Verification items for the finished model (mm, model axes). A direction names the side the tool comes from. Round coordinates to 2 decimals unless told otherwise and drop trailing zeros. Order: outer loops, then holes, each group sorted by start corner. A loop starts at its lowest first (then second) coordinate and runs counter-clockwise, first axis right, second up. Notation, with made-up numbers: (-31, 89) -> (6, 89) arc R11 ccw to (6, 107) -> close; hole circle Ø3 at (26, 63). An arc over 180 degrees is marked (long way). Return JSON: item names as keys, results as strings. Group by question number.
Item 1: Sectioned sample at C-C on z = 11. Record the cut outline in (x, y).
Item 2: Draft check along X on faces 5 (the flat face through (21.431, 0, 0)), 6 (the conical face through (0.16, 1.08, -0.71)), 7 (the cylindrical face through (-8.798, 9.296, -0.133)). Enter one of: pulls with the +X half, pulls with the -X half, needs draft (parallel to the pull), parting line crosses it, or undercut.
Item 3: Sectioned sample at B-B on y = 7.25. Record the cut outline in (x, z).
Item 4: Depth check by flat-ended pin: pin 1 Ø2.5 at (x, y) = (2.5, 9.5) entering from +Z (3 decimals); pin 2 Ø1.4 at (x, y) = (1.5, 11) entering from -Z (3 decimals); pin 3 Ø4 at (x, z) = (1, 12) entering from +Y. Enter the tip coordinate at first touch or a pass-through.
Item 5: Scan lines: probe 1 along Z at (x, y) = (0, -5.25); probe 2 along Z at (x, y) = (0, -10) (3 decimals); probe 3 along X at (y, z) = (-5.5, 0). Record each from-to range of solid material in increasing order. Write a range as from..to.
Item 6: Sectioned sample at A-A on y = 0. Record the cut outline in (x, z), plus the area to 3 significant figures.
Item 7: Sectioned sample at D-D on x = -16. Record the cut outline in (y, z), plus the area to 3 significant figures.
Item 8: Access from +Z, -Z, +X, -X, +Y, -Y to the whole of each face (thin tool, end or side, straight path). Record for faces 1 (the flat face through (0, -10, 9.525)), 2 (the cylindrical face through (0.55, -7.87, 4.18)), 3 (the flat face through (0, 10, 9.525)), 4 (the cylindrical face through (-17.46, 0.07, 18.17)).
```python
from build123d import *

# Parameters (mm, degrees)
SKETCH1_W                   = 42.8625
SKETCH1_H                   = 15.875
EXTRUDE1_DEPTH              = 11.90625
EXTRUDE2_DEPTH              = 9.525
F_3_8_24_TAPPED_HOLE1_D     = 8.4328
F_3_8_24_TAPPED_HOLE1_DEPTH = 9.525
F_3_8_24_TAPPED_HOLE1_TIP   = 2.533468714
F_3_8_24_TAPPED_HOLE2_D     = 8.4328
F_3_8_24_TAPPED_HOLE2_DEPTH = 9.525
F_3_8_24_TAPPED_HOLE2_TIP   = 2.533468714
SKETCH7_R                   = 1.5875
EXTRUDE3_DEPTH              = 12.7


with BuildPart() as part:
    # Sketch1 → Extrude1 (new, symmetric)
    with BuildSketch(Plane.XY):
        Rectangle(SKETCH1_W, SKETCH1_H)
    extrude(amount=EXTRUDE1_DEPTH, both=True)

    # Sketch2 → Extrude2 (add, symmetric)
    with BuildSketch(Plane.XY):
        with BuildLine():
            Line((-7.366, 12.7), (7.366, 12.7))
            ThreePointArc((7.366, 12.7), (8.760903955, 9.332403955), (12.1285, 7.9375))
            Line((12.1285, 7.9375), (-12.1285, 7.9375))
            ThreePointArc((-12.1285, 7.9375), (-8.760903955, 9.332403955), (-7.366, 12.7))
        make_face()
        with BuildLine():
            Line((-7.366, -12.7), (7.366, -12.7))
            ThreePointArc((7.366, -12.7), (8.760903955, -9.332403955), (12.1285, -7.9375))
            Line((12.1285, -7.9375), (-12.1285, -7.9375))
            ThreePointArc((-12.1285, -7.9375), (-8.760903955, -9.332403955), (-7.366, -12.7))
        make_face()
    extrude(amount=EXTRUDE2_DEPTH, both=True)

    # 3/8-24 Tapped Hole1
    with Locations(Plane(origin=(0, 12.7, 0), x_dir=(-1, 0, 0), z_dir=(0, 1, 0))):
        with Locations((0, 0)):
            Hole(F_3_8_24_TAPPED_HOLE1_D / 2, depth=F_3_8_24_TAPPED_HOLE1_DEPTH)
            with Locations((0, 0, -(F_3_8_24_TAPPED_HOLE1_DEPTH + F_3_8_24_TAPPED_HOLE1_TIP / 2))):  # 118° drill point
                Cone(0, F_3_8_24_TAPPED_HOLE1_D / 2, F_3_8_24_TAPPED_HOLE1_TIP, mode=Mode.SUBTRACT)

    # 3/8-24 Tapped Hole2
    with Locations(Plane.XZ.offset(12.7)):
        with Locations((0, 0)):
            Hole(F_3_8_24_TAPPED_HOLE2_D / 2, depth=F_3_8_24_TAPPED_HOLE2_DEPTH)
            with Locations((0, 0, -(F_3_8_24_TAPPED_HOLE2_DEPTH + F_3_8_24_TAPPED_HOLE2_TIP / 2))):  # 118° drill point
                Cone(0, F_3_8_24_TAPPED_HOLE2_D / 2, F_3_8_24_TAPPED_HOLE2_TIP, mode=Mode.SUBTRACT)

    # Sketch7 → Extrude3 (add)
    with BuildSketch(Plane.XY.offset(11.90625)):
        with Locations((-15.875, 0)):
            Circle(SKETCH7_R)
    extrude(amount=EXTRUDE3_DEPTH)


solid = part.part
```
Recorded:
{
 "1": {"outline": "(-21.43, -7.94) -> (21.43, -7.94) -> (21.43, 7.94) -> (-21.43, 7.94) -> close"},
 "2": {"face 5": "pulls with the +X half", "face 6": "undercut", "face 7": "pulls with the -X half"},
 "3": {"outline": "(-21.43, -11.91) -> (21.43, -11.91) -> (21.43, 11.91) -> (-21.43, 11.91) -> close; hole circle Ø8.43 at (0, 0)"},
 "4": {"pin 1": "z = 9.525", "pin 2": "z = -9.525", "pin 3": "y = 7.94"},
 "5": {"probe 1": "-11.91..-4.22, 4.22..11.91", "probe 2": "-9.525..-4.216, 4.216..9.525", "probe 3": "-21.43..-4.22, 4.22..21.43"},
 "6": {"outline": "(-21.43, -11.91) -> (21.43, -11.91) -> (21.43, 11.91) -> (-14.29, 11.91) -> (-14.29, 24.61) -> (-17.46, 24.61) -> (-17.46, 11.91) -> (-21.43, 11.91) -> close", "area": "1,060 mm²"},
 "7": {"outline": "(-7.94, -11.91) -> (7.94, -11.91) -> (7.94, 11.91) -> (1.58, 11.91) -> (1.58, 24.61) -> (-1.58, 24.61) -> (-1.58, 11.91) -> (-7.94, 11.91) -> close", "area": "418 mm²"},
 "8": {"face 1": "+Z, +X, -X, -Y", "face 2": "-Y", "face 3": "+Z, +X, -X, +Y", "face 4": "+Z"}
}
